Could you check a few things on this model? Use its own coordinates, in mm. A direction names the side the tool comes from. Round coordinates to 2 decimals unless told otherwise and drop trailing zeros. Order: outer loops, then holes, each group sorted by start corner. A loop starts at its lowest first (then second) coordinate and runs counter-clockwise, first axis right, second up. Notation, with made-up numbers: (81, 0) - (140, 0) arc R15 cw to (140, 13) - close; hole circle Ø10 at (49.25, 56.25). An arc over 180 degrees is marked (long way). Use one line per item in the form item = value.
from build123d import *

# Parameters (mm, degrees)
SKETCH1_W              = 64.3
SKETCH1_H              = 40.3
BOSS_EXTRUDE1_DEPTH    = 4
SKETCH2_W              = 56
SKETCH2_H              = 33.5
MAIN_WELL_CUTOUT_DEPTH = 3
SKETCH8_R              = 1.27
SKETCH8_W              = 15.536
SKETCH8_H              = 4.826
ADHESIVE_CONTACT_DEPTH = 0.4
SKETCH5_W              = 59.7
SKETCH5_H              = 2.4
CUT_EXTRUDE2_DEPTH     = 2.3
SKETCH5_3_W            = 2.3
SKETCH5_3_H            = 2.4
CUT_EXTRUDE3_DEPTH     = 76.99065732


with BuildPart() as part:
    # Sketch1 → Boss-Extrude1 (new body)
    with BuildSketch(Plane(origin=(0, 0, 0), x_dir=(1, 0, 0), z_dir=(0, 1, 0))):
        with Locations((32.15, 20.15)):
            Rectangle(SKETCH1_W, SKETCH1_H)
    extrude(amount=BOSS_EXTRUDE1_DEPTH)

    # Sketch2 → main well cutout (cut)
    with BuildSketch(Plane(origin=(0, 4, 0), x_dir=(1, 0, 0), z_dir=(0, 1, 0))):
        with Locations((32.15, 20.15)):
            Rectangle(SKETCH2_W, SKETCH2_H)
    extrude(amount=-MAIN_WELL_CUTOUT_DEPTH, mode=Mode.SUBTRACT)

    # Sketch8 → Adhesive contact (add)
    with BuildSketch(Plane(origin=(0, 1, 0), x_dir=(1, 0, 0), z_dir=(0, 1, 0))):
        with Locations(Location((18.374, 32.61, 0), (0, 0, 270))):
            Circle(SKETCH8_R)
        with Locations(Location((18.374, 6.194, 0), (0, 0, 270))):
            Circle(SKETCH8_R)
        with Locations(Location((58.15, 6.194, 0), (0, 0, 270))):
            Circle(SKETCH8_R)
        with Locations(Location((58.15, 32.61, 0), (0, 0, 270))):
            Circle(SKETCH8_R)
        with Locations((41.382, 19.783)):
            Rectangle(SKETCH8_W, SKETCH8_H)
    extrude(amount=ADHESIVE_CONTACT_DEPTH)

    # Sketch5 → Cut-Extrude2 (cut)
    with BuildSketch(Plane.XY):
        with Locations((32.15, 1.2)):
            Rectangle(SKETCH5_W, SKETCH5_H)
    cut_extrude2 = extrude(amount=-CUT_EXTRUDE2_DEPTH, mode=Mode.SUBTRACT)

    # Sketch5_3 → Cut-Extrude3 (cut, through all)
    with BuildSketch(Plane.XY):
        with Locations((1.15, 1.2)):
            Rectangle(SKETCH5_3_W, SKETCH5_3_H)
        with Locations((63.15, 1.2)):
            Rectangle(SKETCH5_3_W, SKETCH5_3_H)
    extrude(amount=-CUT_EXTRUDE3_DEPTH, mode=Mode.SUBTRACT)

    # cuttout mirror: Cut-Extrude2 across plane
    add(cut_extrude2.mirror(Plane.XY.offset(-20.15)), mode=Mode.SUBTRACT)


solid = part.part
Item 1: Imagine slicing it at D-D on x = 58.15. Please give me the cut outline in (y, z).
Found:
outline = (0, -38) - (2.4, -38) - (2.4, -40.3) - (4, -40.3) - (4, -36.9) - (1, -36.9) - (1, -33.88) - (1.4, -33.88) - (1.4, -31.34) - (1, -31.34) - (1, -7.46) - (1.4, -7.46) - (1.4, -4.92) - (1, -4.92) - (1, -3.4) - (4, -3.4) - (4, 0) - (2.4, 0) - (2.4, -2.3) - (0, -2.3) - close
Item 2: I need wall thicknesses on L1, parallel to Z at x = 29, y = 3.15; L2, parallel to X at y = 3.25, z = -18; L3, parallel to Z at x = 37.5, y = 1.9. Which ranges of each line are inside material? Lowest first, please.
Found:
L1 = -40.3 to -36.9, -3.4 to 0
L2 = 0 to 4.15, 60.15 to 64.3
L3 = -38 to -36.9, -3.4 to -2.3
Item 3: Will these pins go through, and if not, where does the flat tip stop? P1, Ø4, axis at x = 39, z = -20, coming from the +Y side; P2, Ø1.2, axis at y = 0.5, z = -19, coming from the -X side; P3, Ø8, axis at x = 21, z = -26, coming from the -Y side; P4, Ø12, axis at x = 22, z = -14.5, coming from the +Y side.
Found:
P1 = 1.4
P2 = 2.3
P3 = 0
P4 = 1
Item 4: Imagine slicing it at C-C on z = -32.61. Please give me the cut outline in (x, y).
Found:
outline = (0, 2.4) - (2.3, 2.4) - (2.3, 0) - (62, 0) - (62, 2.4) - (64.3, 2.4) - (64.3, 4) - (60.15, 4) - (60.15, 1) - (59.42, 1) - (59.42, 1.4) - (56.88, 1.4) - (56.88, 1) - (19.64, 1) - (19.64, 1.4) - (17.1, 1.4) - (17.1, 1) - (4.15, 1) - (4.15, 4) - (0, 4) - close
Item 5: For faces 1 (the face through (2.3, 1, -20)), 2 (the face through (32, 1, -38)), 3 (the face through (41, 1.4, -20)), which set-ups out of +Z, -Z, +X, -X, +Y, -Y let a thin tool reach every point of the face, with its end or its side?
Found:
face_1 = +Z, -Z, -X, -Y
face_2 = -Z, +X, -X, -Y
face_3 = +Y
Item 6: Imagine slicing it at A-A on y = 3.4. Please give me the cut outline in (x, z), plus the area to 3 significant figures.
Found:
outline = (0, -40.3) - (64.3, -40.3) - (64.3, 0) - (0, 0) - close; hole (4.15, -36.9) - (60.15, -36.9) - (60.15, -3.4) - (4.15, -3.4) - close
area = 715 mm2
Item 7: Imagine slicing it at B-B on x = 13.5. Please give me the cut outline in (y, z), plus the area to 3 significant figures.
Found:
outline = (0, -38) - (2.4, -38) - (2.4, -40.3) - (4, -40.3) - (4, -36.9) - (1, -36.9) - (1, -3.4) - (4, -3.4) - (4, 0) - (2.4, 0) - (2.4, -2.3) - (0, -2.3) - close
area = 49.7 mm2
Item 8: If we mould it in two halves opening along X, with no side actions, what happens to faces 4 (the face through (4.15, 3, -20)), 5 (the face through (62, 1, -20)), 6 (the face through (32, 0, -20))? For each: released by +X, released by -X, zero draft, split by the parting line, or undercut.
Found:
face_4 = undercut
face_5 = released by +X
face_6 = zero draft
